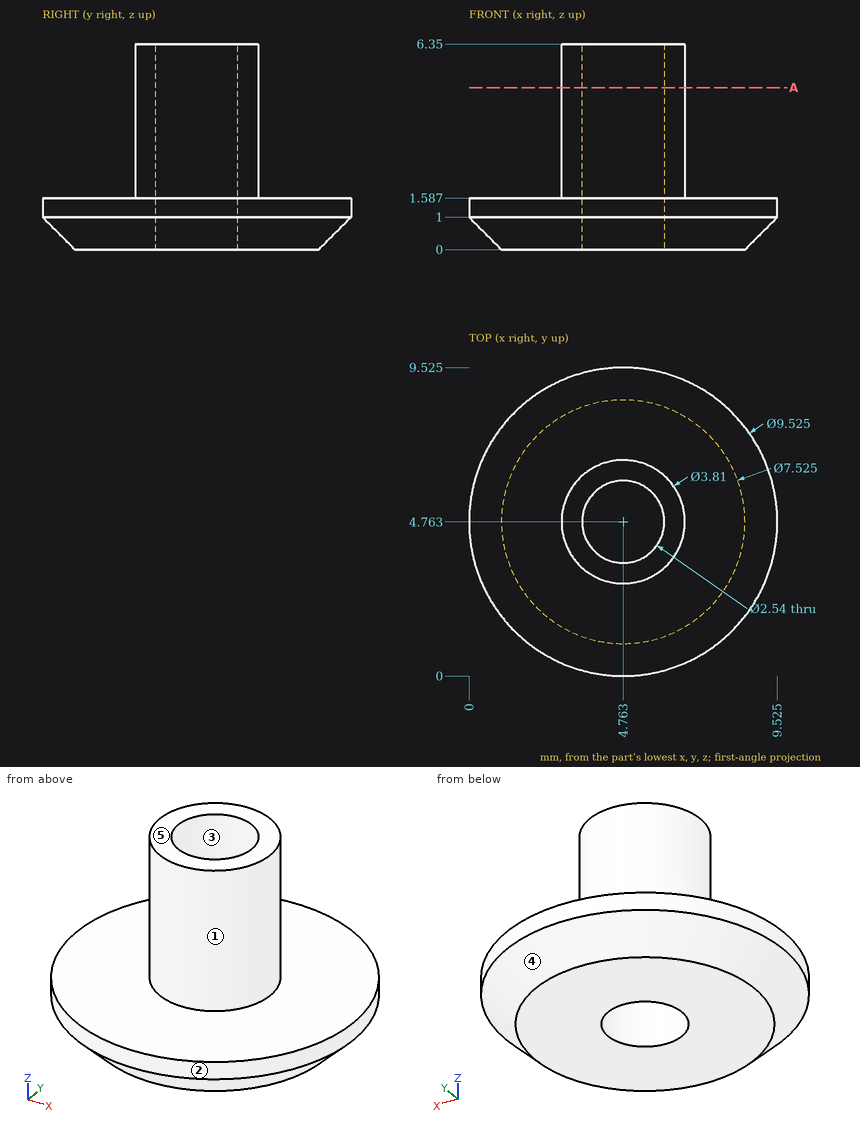
Geometry: see drawing. Coordinates: mm, zero at the bounding-box minimum. A direction names the side the tool comes from. Coordinates: 2 decimals unless noted, no trailing zeros. Order: outer loops, then holes, each group sorted by start corner. A loop starts at its lowest first (then second) coordinate and runs counter-clockwise, first axis right, second up. Notation, with made-up numbers: (4, 77.5) - (31, 77.5) arc R23 ccw to (31, 97.5) - close; hole circle Ø1 at (5.5, 65.5). An arc over 180 degrees is marked (long way). Return JSON: item names as keys, results as strings.
Q1. Access query for the marked faces 1 and 2. Directions: +Z, -Z, +X, -X, +Y, -Y. A direction counts if a zero-diameter tool reaches every point of the face in a straight line with its end or side. Return the directions, or none.
The answers:
{"face 1": "+Z", "face 2": "+Z, -Z"}
Q2. First-contact query: pin 1 (1.5 mm diameter, centred on y = 7.5, z = 5, fed in from +X). Flat tip, straight axial feed; report the tip coordinate or a pass-through.
The answers:
{"pin 1": "passes through"}
Q3. Cut plane A-A (z = 5). Return loops of the section in (x, y) (1 decimal).
The answers:
{"outline": "circle Ø3.8 at (4.8, 4.8); hole circle Ø2.5 at (4.8, 4.8)"}
Q4. Ray query, probe 1 along Z at (x, y) = (7.5, 3.75); probe 2 along Y at (x, z) = (4, 2.75) (1 decimal); probe 3 along X at (y, z) = (9, 1.5) (1 decimal). Return the intervals inside material, ascending.
The answers:
{"probe 1": "z = 0 to 1.59", "probe 2": "y = 3 to 3.7, 5.8 to 6.5", "probe 3": "x = 2.6 to 6.9"}
Q5. Draft query along X for the marked faces 3, 4 and 5. Return one class per face: +X half, -X half, draft (parallel to the pull), parting line (faces both ways), or undercut.
The answers:
{"face 3": "undercut", "face 4": "parting line", "face 5": "draft"}
